Geometry check sheet. Reference: the model listing, model coordinates, mm. Face numbers are marked on the shaded views. A direction names the side the tool comes from. Coordinates: 2 decimals unless noted, no trailing zeros. Write each loop counter-clockwise with the first axis right and the second up, starting at its lowest first coordinate (ties: lowest second). Pieces come first, ordered by that corner, then holes. Notation, with made-up numbers: (54.25, 82.5) -> (96.25, 82.5) arc R13 ccw to (96.25, 94.5) -> close; hole circle Ø6 at (84.25, -6). An arc over 180 degrees is marked (long way). Answer in a Markdown table with one row per item. Add a question column.
Q1. Tool access check on the marked faces 1, 2, 3, 4 and 5. Record the directions out of +Z, -Z, +X, -X, +Y, -Y that give a thin tool (end or side, any length) a straight path to the whole face; none if there is none.
Q2. Section check A-A, the plane x = -1. Record the boundary of the cut face in (y, z).
Q3. Thickness scan on line 1 (Y direction, x = -9, z = 3.25); line 2 (Y direction, x = 53, z = 2.75); line 3 (X direction, y = -120.5, z = 0.5). Record the ranges inside material, lowest first.
Q4. Gauge pin test, flat ends, axial feed: P1, Ø1.1, axis at x = 5, z = 6.5, coming from the +Y side; P2, Ø2, axis at x = 55.5, z = 2, coming from the -Y side; P3, Ø1.4, axis at x = -29.02, y = -86.93, coming from the +Z side; P4, Ø1.5, axis at y = -132, z = 1.5, coming from the -X side. Record the tip position at first contact, or that the pin passes through.
```python
from build123d import *

# Parameters (mm, degrees)
ESBO_O1_W                = 56
ESBO_O1_H                = 30
ESBO_O1_W_2              = 100
ESBO_O1_H_2              = 45
RESSALTO_EXTRUS_O1_DEPTH = 7
CORTE_EXTRUS_O1_DEPTH    = 176.483223745
CORTE_EXTRUS_O2_DEPTH    = 164.946216229
ESBO_O5_W                = 17
ESBO_O5_H                = 10
CORTE_EXTRUS_O4_DEPTH    = 3.5
CORTE_EXTRUS_O6_DEPTH    = 24
FILETE1_R                = 2
FILETE2_R                = 2
ESBO_O8_R                = 0.8
ESBO_O8_W                = 6
ESBO_O8_H                = 9
CORTE_EXTRUS_O7_DEPTH    = 24
FILETE3_R                = 2
ESBO_O9_W                = 56
ESBO_O9_H                = 15
CORTE_EXTRUS_O8_DEPTH    = 1
ESBO_O10_R               = 1.45
CORTE_EXTRUS_O9_DEPTH    = 17
ESBO_O11_R               = 2
CORTE_EXTRUS_O10_DEPTH   = 15
CHANFRO1_SIZE            = 2
ESBO_O12_R               = 1.45
CORTE_EXTRUS_O11_DEPTH   = 15


with BuildPart() as part:
    # Esboço1 → Ressalto-extrusão1 (new body)
    with BuildSketch(Plane.XY):
        with Locations((15.481715893, -129.032502637)):
            Rectangle(ESBO_O1_W, ESBO_O1_H)
        with Locations((15.481715893, -91.532502637)):
            Rectangle(ESBO_O1_W_2, ESBO_O1_H_2)
    extrude(amount=RESSALTO_EXTRUS_O1_DEPTH)

    # Esboço2 → Corte-extrusão1 (cut, through all)
    with BuildSketch(Plane.ZY.offset(34.518284107)):
        Polygon((0.6, -69.032502637), (7, -69.032502637), (7, -80.532502637), (3.876629102, -78.564484615), (2.702851981, -78.813978644), align=None)
    extrude(amount=-CORTE_EXTRUS_O1_DEPTH, mode=Mode.SUBTRACT)

    # Esboço3 → Corte-extrusão2 (cut, through all)
    with BuildSketch(Plane(origin=(43.481715893, 0, 0), x_dir=(0, 0, -1), z_dir=(1, 0, 0))):
        Polygon((-5, -144.032502637), (0, -139.032502637), (0, -144.032502637), align=None)
    extrude(amount=-CORTE_EXTRUS_O2_DEPTH, mode=Mode.SUBTRACT)

    # Esboço5 → Corte-extrusão4 (cut)
    with BuildSketch(Plane.XY.offset(7)):
        with Locations((-24.018284107, -86.931905633)):
            Rectangle(ESBO_O5_W, ESBO_O5_H)
        with Locations((54.981715893, -86.931905633)):
            Rectangle(ESBO_O5_W, ESBO_O5_H)
    extrude(amount=-CORTE_EXTRUS_O4_DEPTH, mode=Mode.SUBTRACT)

    # Esboço7 → Corte-extrusão6 (cut)
    with BuildSketch(Plane.XY.offset(7)):
        Polygon((64.477557131, -69.032502637), (65.481715893, -69.032502637), (65.481715893, -78.564484615), align=None)
        Polygon((-34.518284107, -78.564484615), (-33.514125345, -69.032502637), (-34.518284107, -69.032502637), align=None)
    extrude(amount=-CORTE_EXTRUS_O6_DEPTH, mode=Mode.SUBTRACT)

    # Filete1
    filete1_edges = [part.edges().sort_by_distance(p)[0] for p in [
        (-32.518284107, -91.931905633, 5.25),
        (-32.518284107, -81.931905633, 5.25),
        (-15.518284107, -81.931905633, 5.25),
        (-15.518284107, -91.931905633, 5.25),
        (46.481715893, -91.931905633, 5.25),
        (46.481715893, -81.931905633, 5.25),
        (63.481715893, -81.931905633, 5.25),
        (63.481715893, -91.931905633, 5.25),
    ]]
    fillet(filete1_edges, radius=FILETE1_R)

    # Filete2
    filete2_edges = [part.edges().sort_by_distance(p)[0] for p in [
        (-12.518284107, -114.032502637, 3.5),
        (43.481715893, -114.032502637, 3.5),
    ]]
    fillet(filete2_edges, radius=FILETE2_R)

    # Esboço8 → Corte-extrusão7 (cut)
    with BuildSketch(Plane.XY.offset(7)):
        with Locations((59.981716293, -86.931906013)):
            Circle(ESBO_O8_R)
        with Locations((-29.018284507, -86.931905253)):
            Circle(ESBO_O8_R)
        with Locations((-24.518284107, -86.931905633)):
            Rectangle(ESBO_O8_W, ESBO_O8_H)
        with Locations((55.481715893, -86.931905633)):
            Rectangle(ESBO_O8_W, ESBO_O8_H)
    extrude(amount=-CORTE_EXTRUS_O7_DEPTH, mode=Mode.SUBTRACT)

    # Filete3
    filete3_edges = [part.edges().sort_by_distance(p)[0] for p in [
        (-27.518284107, -91.431905633, 1.75),
        (-27.518284107, -82.431905633, 1.75),
        (-21.518284107, -82.431905633, 1.75),
        (-21.518284107, -91.431905633, 1.75),
        (52.481715893, -91.431905633, 1.75),
        (52.481715893, -82.431905633, 1.75),
        (58.481715893, -82.431905633, 1.75),
        (58.481715893, -91.431905633, 1.75),
    ]]
    fillet(filete3_edges, radius=FILETE3_R)

    # Esboço9 → Corte-extrusão8 (cut)
    with BuildSketch(Plane.XY.offset(7)):
        with Locations((15.481715893, -131.532502637)):
            Rectangle(ESBO_O9_W, ESBO_O9_H)
    extrude(amount=-CORTE_EXTRUS_O8_DEPTH, mode=Mode.SUBTRACT)

    # Esboço10 → Corte-extrusão9 (cut)
    with BuildSketch(Plane.XY.offset(7)):
        with Locations((-3.768284107, -119.906030775)):
            Circle(ESBO_O10_R)
        with Locations((34.731715893, -119.906030775)):
            Circle(ESBO_O10_R)
        with Locations((34.731715893, -141.457502637)):
            Circle(ESBO_O10_R)
        with Locations((-3.768284107, -141.457502637)):
            Circle(ESBO_O10_R)
    extrude(amount=-CORTE_EXTRUS_O9_DEPTH, mode=Mode.SUBTRACT)

    # Esboço11 → Corte-extrusão10 (cut)
    with BuildSketch(Plane(origin=(0, 0, 0), x_dir=(-1, 0, 0), z_dir=(0, 0, -1))):
        with Locations((-40.481715893, -86.292423409)):
            Circle(ESBO_O11_R)
        with Locations((9.518284107, -86.292423409)):
            Circle(ESBO_O11_R)
    extrude(amount=-CORTE_EXTRUS_O10_DEPTH, mode=Mode.SUBTRACT)

    # Chanfro1
    chanfro1_edges = [part.edges().sort_by_distance(p)[0] for p in [
        (42.481715893, -86.292423409, 0),
        (-7.518284107, -86.292423409, 0),
    ]]
    chamfer(chanfro1_edges, length=CHANFRO1_SIZE)

    # Esboço12 → Corte-extrusão11 (cut)
    with BuildSketch(Plane(origin=(0, 0, 0), x_dir=(-1, 0, 0), z_dir=(0, 0, -1))):
        with Locations((-59.431715893, -110.532502637)):
            Circle(ESBO_O12_R)
        with Locations((28.468284107, -110.532502637)):
            Circle(ESBO_O12_R)
    extrude(amount=-CORTE_EXTRUS_O11_DEPTH, mode=Mode.SUBTRACT)


solid = part.part
```
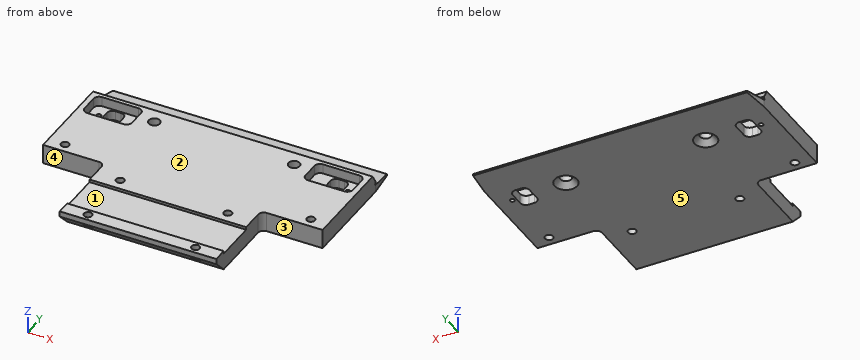
Calculated:
| question | item | result |
|---|---|---|
| 1 | face 1 | +Z, +X, -X |
| 1 | face 2 | +Z, +X, -X, +Y, -Y |
| 1 | face 3 | +Z, -Z, +X, -Y |
| 1 | face 4 | +Z, -Z, -X, -Y |
| 1 | face 5 | -Z, +X, -X, +Y, -Y |
| 2 | outline | (-144.03, 5) -> (-139.03, 0) -> (-69.03, 0) -> (-69.03, 0.6) -> (-78.81, 2.7) -> (-78.56, 3.88) -> (-80.53, 7) -> (-124.03, 7) -> (-124.03, 6) -> (-139.03, 6) -> (-139.03, 7) -> (-144.03, 7) -> close |
| 3 | line 1 | y = -142.28 to -88.22, -84.36 to -78.7 |
| 3 | line 2 | y = -114.03 to -90.78, -83.09 to -78.8 |
| 3 | line 3 | x = -12.52 to -5.09, -2.45 to 33.41, 36.05 to 43.48 |
| 4 | P1 | stops at y = -79.87 |
| 4 | P2 | stops at y = -114.03 |
| 4 | P3 | passes through |
| 4 | P4 | stops at x = -12.52 |
